Can you work these out from the model? Positions are in its coordinate system, mm. A direction names the side the tool comes from. Give positions to 0.01 mm unless a question says otherwise; leave off trailing zeros. Loops run counter-clockwise (first coordinate to the right, second up) from the corner with the lowest first, then second, coordinate; pieces in that order, holes last. Notation, with made-up numbers: (0.5, 43.25) - (55.5, 43.25) arc R12 ccw to (55.5, 59.25) - close; hole circle Ø3 at (7.5, 64). An arc over 180 degrees is marked (long way). Answer in a Markdown table with one row per item.
Autodesk Inventor part; units mm, degrees
ref_plane "YZ Plane" through (0, 0, 0) normal (1, 0, 0) x (0, 1, 0)
ref_plane "XZ Plane" through (0, 0, 0) normal (0, 1, 0) x (-1, 0, 0)
ref_plane "XY Plane" through (0, 0, 0) normal (0, 0, 1) x (1, 0, 0)
ref_plane "РабПлоскость2" through (19.838, 4.4675, -12.3) normal (0, 0, 1) x (1, 0, 0)
ref_plane "РабПлоскость1" through (-13.412, 18.3334, -19.05) normal (0, 0, 1) x (1, 0, 0)
sketch "Эскиз1" plane through (19.838, 4.4675, -12.3) normal (0, 0, 1) x (1, 0, 0)
  line L0 (-17.838, -7.8158) -> (-21.838, -7.8158)
  line L1 (-21.838, -12.9158) -> (-17.838, -12.9158)
  line L2 (-15.838, -12.5585) -> (-15.838, -8.173)
  line L3 (-23.838, -12.5585) -> (-23.838, -8.173)
  line L4 (-15.688, -12.9158) -> (-23.988, -12.9158)
  line L5 (-23.988, -12.9158) -> (-23.988, -7.5158)
  line L6 (-23.988, -7.5158) -> (-15.688, -7.5158)
  line L7 (-15.688, -7.5158) -> (-15.688, -12.9158)
  line L8 (-15.688, -12.9158) -> (-23.988, -7.5158) construction
  line L9 (-19.838, -4.4675) -> (-19.838, -10.2158) construction
  line L10 (-15.388, -12.9158) -> (-24.288, -12.9158)
  line L11 (-6.75, -10.8528) -> (-33.25, -10.8528)
  line L12 (-33.25, -10.8528) -> (-6.75, -10.8528)
  line L13 (-33.25, -10.8528) -> (-6.75, -10.8528) construction
  line L14 (-24.938, -14.0158) -> (-14.738, -14.0158)
  line L15 (-15.388, -12.9158) -> (-24.288, -12.9158)
  line L16 (-19.838, -14.0158) -> (-19.838, -12.9158) construction
  line L17 (-13.838, -13.4658) -> (-25.838, -13.4658) construction
  line L18 (-25.838, -13.4658) -> (-25.838, -3.5158)
  line L19 (-25.838, -3.5158) -> (-13.838, -3.5158)
  line L20 (-13.838, -3.5158) -> (-13.838, -13.4658)
  line L21 (-6.75, -10.8528) -> (-33.25, -10.8528)
  line L22 (-33.25, -10.8528) -> (-33.25, -3.5158) construction
  line L23 (-33.25, -3.5158) -> (-6.75, -3.5158)
  line L24 (-6.75, -3.5158) -> (-6.75, -10.8528) construction
  line L25 (-6.75, -3.5158) -> (-6.75, -1.5158) construction
  line L26 (-33.25, -3.5158) -> (-33.25, -1.5158) construction
  arc A0 (-33.25, -1.5158) -> (-6.75, -1.5158) centre (-20, 41.3683) ccw
  line L27 (-25.838, -13.4658) -> (-13.838, -13.4658) construction
  line L28 (-13.838, -13.4658) -> (-25.838, -13.4658)
  line L29 (-4.75, -0.8459) -> (-4.75, -27.8528)
  line L30 (-35.25, -0.8459) -> (-35.25, -27.8528)
  arc A1 (-35.25, -0.8459) -> (-33.25, -1.5158) centre (-20, 41.3683) ccw
  arc A2 (-6.75, -1.5158) -> (-4.75, -0.8459) centre (-20, 41.3683) ccw
  line L31 (-33.25, -14.9158) -> (-33.25, -27.8528)
  line L32 (-33.25, -27.8528) -> (-35.25, -27.8528)
  line L33 (-6.75, -14.9158) -> (-6.75, -27.8528)
  line L34 (-6.75, -27.8528) -> (-4.75, -27.8528)
  line L35 (-33.25, -14.9158) -> (-6.75, -14.9158)
  point P0 (-19.838, -13.4658)
  point P1 (-19.838, -3.5158)
  point P2 (-25.838, -10.8528)
  point P3 (-13.838, -10.8528)
  point P4 (-20.162, -3.5158)
  point P5 (-15.688, -10.8528)
  point P6 (-23.988, -10.8528)
  point P7 (-20.162, -3.5158)
  point P8 (-17.838, -12.9158)
  dimension "d0" = 8.3
  dimension "d1" = 5.4
  dimension "d2" = 12
  dimension "d3" = 4
  dimension "d4" = 2
  dimension "d10" = 0
  dimension "d11" = 0.55
  dimension "d26" = 2
  dimension "d27" = 2
  dimension "d30" = 17
  dimension "d33" = 2
extrude "Выдавливание1" add sketch "Эскиз1" along normal mid plane 11.5 contours L4 L5 L11 L7 L1 | L1 L4 L7 L11 L20 L28 L18 L5 | L11 L18 L19 L20 L7 L6 L5 | L5 L6 L7 L11 | A0 A2 L29 L34 L33 L35 L31 L32 L30 A1
sketch "Эскиз3" plane through (-6, -10.4482, -6.55) normal (0, -1, 0) x (1, 0, 0)
  circle A0 centre (5.838, -5.75) radius 2
  line L0 (19.088, -11.5) -> (19.088, 0)
  line L1 (-7.412, -11.5) -> (-7.412, 0)
  line L2 (-7.412, 0) -> (19.088, -11.5) construction
  line L3 (5.838, 12.0241) -> (5.838, -23.5241) construction
  line L4 (-15.512, -5.75) -> (27.188, -5.75) construction
  line L5 (2.288, -3.7004) -> (5.838, -1.6508)
  line L6 (5.838, -1.6508) -> (9.388, -3.7004)
  line L7 (9.388, -3.7004) -> (9.388, -7.7996)
  line L8 (9.388, -7.7996) -> (5.838, -9.8492) construction
  line L9 (5.838, -9.8492) -> (2.288, -7.7996) construction
  line L10 (2.288, -7.7996) -> (2.288, -3.7004)
  line L11 (2.288, -7.7996) -> (2.288, -12.2488)
  line L12 (9.388, -7.7996) -> (9.388, -11.5)
  line L13 (19.088, -11.5) -> (-7.412, -11.5)
  point P0 (6, 6.55)
  point P1 (0, 0)
  point P2 (12, -12.8)
  point P3 (2.288, -5.75)
  point P4 (2.288, -11.5)
  dimension "d12" = 4
  dimension "d34" = 3.55
extrude "Выдавливание8" cut sketch "Эскиз3" against normal blind 5.3 contours A0 | L5 L6 L7 L12 L13 L11 L10
extrude "Выдавливание9" add sketch "Эскиз3" against normal blind 2
extrude "Выдавливание10" cut sketch "Эскиз3" against normal blind 9 contours A0
fillet "Сопряжение1" radius 1.5 2 edges at (-15.412, 3.6216, -12.3) (15.088, 3.6216, -12.3)
equation "\"d27\" = d26"
properties part number "kicker1.1"
Q1. For pin 1 (2 mm diameter, centred on x = 0, z = -14, fed in from +Y); pin 2 (6 mm diameter, centred on x = -9.5, z = -8.5, fed in from +Y); pin 3 (3 mm diameter, centred on x = -0.5, z = -12, fed in from -Y); pin 4 (6 mm diameter, centred on x = -8.5, y = -14.5, fed in from -Z), each with a flat end and sliding along its axis, tell me the tip position at first contact or that it passes through.
Checked values:
| item | result |
|---|---|
| pin 1 | stops at y = 0.97 |
| pin 2 | stops at y = 2.68 |
| pin 3 | stops at y = -1.45 |
| pin 4 | passes through |
Q2. Imagine slicing it at B-B, the plane z = -15.25. Write out the boundary of the cut face in (x, y).
Checked values:
| item | result |
|---|---|
| outline | (-15.41, -23.39) - (-13.41, -23.39) - (-13.41, -10.45) - (3.39, -10.45) - (13.09, -10.45) - (13.09, -23.39) - (15.09, -23.39) - (15.09, 1.54) arc R1.5 ccw to (13.14, 2.97) arc R44.74 cw to (13.09, 2.95) arc R44.88 cw to (-13.41, 2.95) arc R45.03 cw to (-13.47, 2.97) arc R1.5 ccw to (-15.41, 1.54) - close; hole (-3.71, -8.45) - (3.39, -8.45) - (3.39, -5.15) - (-3.71, -5.15) - close |
Q3. Imagine slicing it at D-D, the plane z = -7.75. Write out the boundary of the cut face in (x, y).
Checked values:
| item | result |
|---|---|
| outline | (-15.41, -23.39) - (-13.41, -23.39) - (-13.41, -10.45) - (13.09, -10.45) - (13.09, -23.39) - (15.09, -23.39) - (15.09, 1.54) arc R1.5 ccw to (13.14, 2.97) arc R44.74 cw to (13.09, 2.95) arc R44.88 cw to (-13.41, 2.95) arc R45.03 cw to (-13.47, 2.97) arc R1.5 ccw to (-15.41, 1.54) - close |
Q4. Imagine slicing it at A-A, the plane y = -16.5. Write out the boundary of the cut face in (x, z), and give its area (3 significant figures).
Checked values:
| item | result |
|---|---|
| outline | (-15.41, -18.05) - (-13.41, -18.05) - (-13.41, -6.55) - (-15.41, -6.55) - close; (13.09, -18.05) - (15.09, -18.05) - (15.09, -6.55) - (13.09, -6.55) - close |
| area | 46.0 mm² |
Q5. If we mould it in two halves opening along X, with no side actions, what happens to faces 1 (the face through (13.088, -17, -12)), 2 (the face through (0, -7, -6.55)), 3 (the face through (15.088, -11, -12)), 4 (the face through (0.03, 0.95, -12.38))? For each: released by +X, released by -X, zero draft, split by the parting line, or undercut.
Checked values:
| item | result |
|---|---|
| face 1 | undercut |
| face 2 | zero draft |
| face 3 | released by +X |
| face 4 | undercut |
Q6. On a 3-axis mill with a long thin cutter (end or side, diameter ignored), from which of +Z, -Z, +X, -X, +Y, -Y can I reach the whole of each face in a straight line? I mean faces 5 (the face through (0, -8.448, -15)), 6 (the face through (-13.412, -17, -12)), 7 (the face through (0, -1.448, -12)). Say none if no direction works.
Checked values:
| item | result |
|---|---|
| face 5 | -Z |
| face 6 | +Z, -Z, -Y |
| face 7 | -Y |
Q7. If I drill on line 1 (X direction, y = -12.5, z = -12); line 2 (X direction, y = -6.75, z = -16); line 3 (Y direction, x = 7, z = -16.75), over which ranges is the centre line in solid material (lowest first)? Write a range as [from, to].
Checked values:
| item | result |
|---|---|
| line 1 | x = [-15.41, -13.41], [13.09, 15.09] |
| line 2 | x = [-15.41, -3.71], [3.39, 15.09] |
| line 3 | y = [-10.45, 1.53] |
Q8. Imagine slicing it at C-C, the plane z = -12.3. Write out the boundary of the cut face in (x, y).
Checked values:
| item | result |
|---|---|
| outline | (-15.41, -23.39) - (-13.41, -23.39) - (-13.41, -10.45) - (-2.16, -10.45) - (-2.16, -8.45) - (-3.71, -8.45) - (-3.71, -5.15) - (-2.16, -5.15) - (-2.16, -1.45) - (1.84, -1.45) - (1.84, -5.15) - (3.39, -5.15) - (3.39, -8.45) - (1.84, -8.45) - (1.84, -10.45) - (13.09, -10.45) - (13.09, -23.39) - (15.09, -23.39) - (15.09, 1.54) arc R1.5 ccw to (13.14, 2.97) arc R44.74 cw to (13.09, 2.95) arc R44.88 cw to (-13.41, 2.95) arc R45.03 cw to (-13.47, 2.97) arc R1.5 ccw to (-15.41, 1.54) - close |
